Design review of the part shown in the three views and the two pictorial views. Dimensions are in mm from the part's minimum x, y and z. A direction names the side the tool comes from. Give positions to 0.01 mm unless a question says otherwise; leave off trailing zeros. Order: outer loops, then holes, each group sorted by start corner. A loop starts at its lowest first (then second) coordinate and runs counter-clockwise, first axis right, second up.
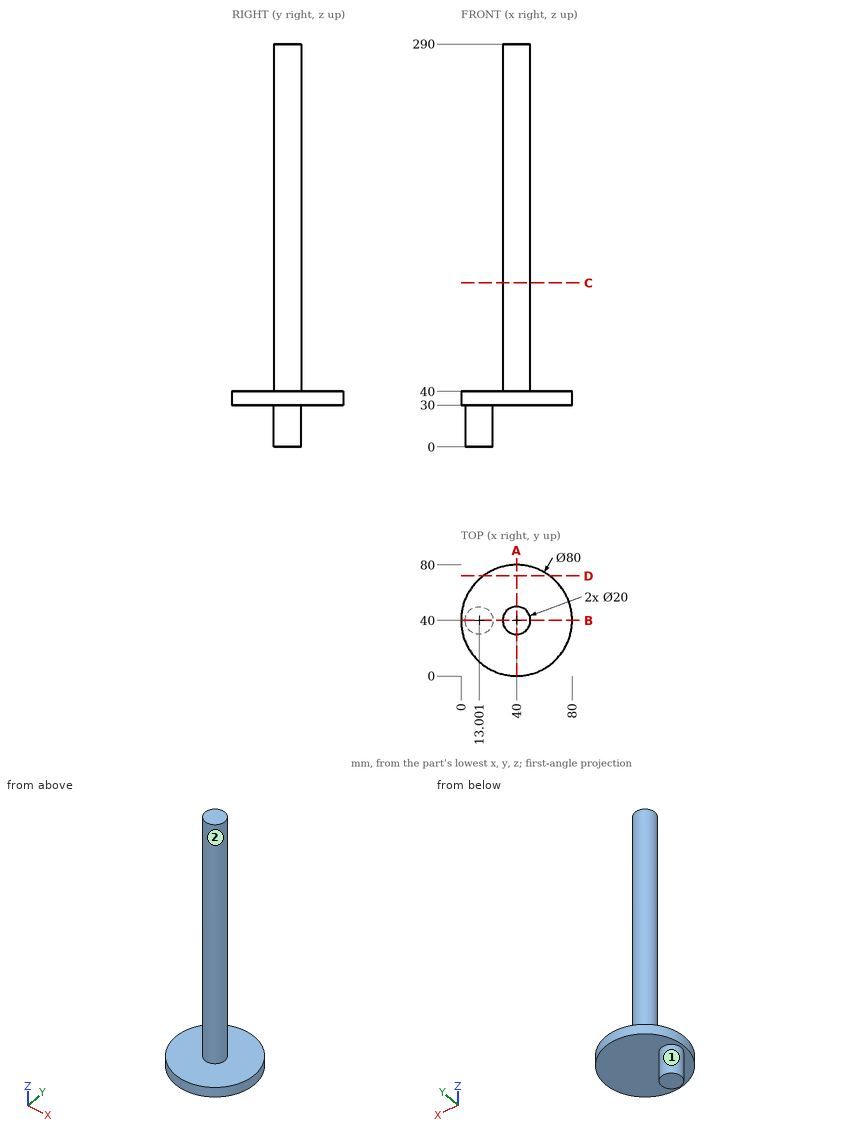
Item 1: For the marked faces 1 and 2, list the 3-axis set-ups (+Z, -Z, +X, -X, +Y, -Y) from which the entire face can be reached by the end or side of a thin tool; tool diameter is ignored.
Values found:
face 1: -Z
face 2: +Z
Item 2: Take a section at A-A (x = 40). Give the boundary of the cut face in (y, z), and give its area (3 significant figures).
Values found:
outline: (0, 30) - (80, 30) - (80, 40) - (50, 40) - (50, 290) - (30, 290) - (30, 40) - (0, 40) - close
area: 5,800 mm2
Item 3: Take a section at B-B (y = 40). Give the boundary of the cut face in (x, z), and give its area (3 significant figures).
Values found:
outline: (0, 30) - (3, 30) - (3, 0) - (23, 0) - (23, 30) - (80, 30) - (80, 40) - (50, 40) - (50, 290) - (30, 290) - (30, 40) - (0, 40) - close
area: 6,400 mm2
Item 4: Take a section at C-C (z = 118). Give the boundary of the cut face in (x, y), and give its area (3 significant figures).
Values found:
outline: circle Ø20 at (40, 40)
area: 314 mm2
Item 5: Take a section at D-D (y = 72). Give the boundary of the cut face in (x, z).
Values found:
outline: (16, 30) - (64, 30) - (64, 40) - (16, 40) - close
Item 6: For line 1 (Z direction, x = 40.5, y = 74); line 2 (X direction, y = 39, z = 94), list the stretches that pass through material, from the lowest coordinate up.
Values found:
line 1: z = 30 to 40
line 2: x = 30.05 to 49.95
Item 7: Clearance check with flat-ended pins moving along their axes: pin 1 Ø12 at (x, y) = (51, 9.5) entering from +Z; pin 2 Ø3 at (y, z) = (30, 124) entering from +X; pin 3 Ø8 at (x, z) = (39.5, 225.5) entering from -Y. State where each tip first meets the part, or that it passes through.
Values found:
pin 1: stops at z = 40
pin 2: stops at x = 45.27
pin 3: stops at y = 30
